Could you check a few things on this model? Use its own coordinates, in mm. Coordinates: 2 decimals unless noted, no trailing zeros. Write each loop counter-clockwise with the first axis right and the second up, starting at its lowest first coordinate (ties: lowest second). Pieces come first, ordered by that corner, then holes.
Item 1: I want a section at C-C on x = -134. Please give me the cut outline in (y, z) (3 decimals), then the cut area to 4 significant figures.
Item 2: For P1, Ø5.5, axis at x = -134, y = 105, coming from the -Z side, with a flat end and sliding along its axis, tell me the tip position at first contact or that it passes through.
Item 3: I want a section at A-A on y = 80. Please give me the cut outline in (x, z) (3 decimals), then the cut area to 4 significant figures.
Item 4: If I drill on probe 1 along X at (y, z) = (28, 0.35); probe 2 along Y at (x, z) = (-5, 0.35) (3 decimals); probe 3 along X at (y, z) = (29, 0.15), over which ranges is the centre line in solid material (lowest first)?
Item 5: I want a section at B-B on z = 0.2. State how many separate pieces and enclosed holes the cut face has, then the cut area to 3 significant figures.
from build123d import *

# Parameters (mm, degrees)
RESSALTO_EXTRUS_O1_DEPTH                       = 0.5
BROCA_DE_ROSQUEAR_PARA_TARRAXA_DE_M3X0_5_D     = 6.35
BROCA_DE_ROSQUEAR_PARA_TARRAXA_DE_M3X0_5_DEPTH = 23.492267535
BROCA_DE_ROSQUEAR_PARA_TARRAXA_DE_M3X0_5_TIP   = 1.907732465


with BuildPart() as part:
    # Esboço1 → Ressalto-extrusão1 (new body)
    with BuildSketch(Plane.XY):
        with BuildLine():
            Line((-10, 0), (-164, 0))
            ThreePointArc((-164, 0), (-171.071067812, 2.928932188), (-174, 10))
            Line((-174, 10), (-174, 100))
            ThreePointArc((-174, 100), (-171.071067812, 107.071067812), (-164, 110))
            Line((-164, 110), (-10, 110))
            ThreePointArc((-10, 110), (-2.928932188, 107.071067812), (0, 100))
            Line((0, 100), (0, 10))
            ThreePointArc((0, 10), (-2.928932188, 2.928932188), (-10, 0))
        make_face()
    extrude(amount=RESSALTO_EXTRUS_O1_DEPTH)

    # Broca de rosquear para tarraxa de M3x0.51
    with Locations(Plane.XY.offset(0.5)):
        with Locations((-169, 80), (-134, 105), (-40, 105), (-5, 80), (-5, 30), (-169, 30), (-134, 5), (-40, 5)):
            Hole(BROCA_DE_ROSQUEAR_PARA_TARRAXA_DE_M3X0_5_D / 2, depth=BROCA_DE_ROSQUEAR_PARA_TARRAXA_DE_M3X0_5_DEPTH)
            with Locations((0, 0, -(BROCA_DE_ROSQUEAR_PARA_TARRAXA_DE_M3X0_5_DEPTH + BROCA_DE_ROSQUEAR_PARA_TARRAXA_DE_M3X0_5_TIP / 2))):  # 118° drill point
                Cone(0, BROCA_DE_ROSQUEAR_PARA_TARRAXA_DE_M3X0_5_D / 2, BROCA_DE_ROSQUEAR_PARA_TARRAXA_DE_M3X0_5_TIP, mode=Mode.SUBTRACT)


solid = part.part
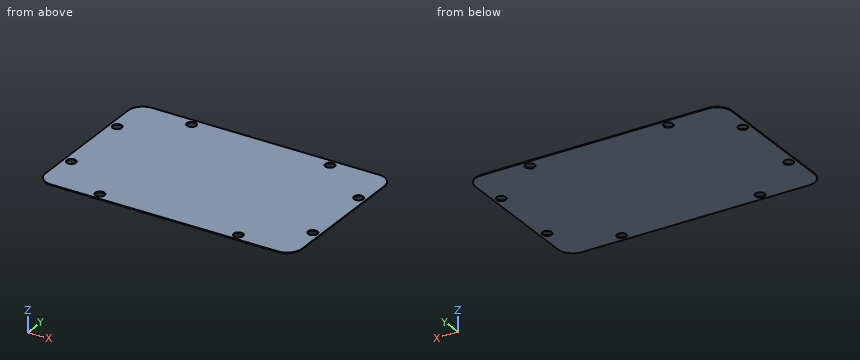
Response values:
1. outline: (0, 0) - (1.825, 0) - (1.825, 0.5) - (0, 0.5) - close; (8.175, 0) - (101.825, 0) - (101.825, 0.5) - (8.175, 0.5) - close; (108.175, 0) - (110, 0) - (110, 0.5) - (108.175, 0.5) - close
1. area: 48.65 mm2
2. P1: passes through
3. outline: (-174, 0) - (-172.175, 0) - (-172.175, 0.5) - (-174, 0.5) - close; (-165.825, 0) - (-8.175, 0) - (-8.175, 0.5) - (-165.825, 0.5) - close; (-1.825, 0) - (0, 0) - (0, 0.5) - (-1.825, 0.5) - close
3. area: 80.65 mm2
4. probe 1: x = -174 to -171.47, -166.53 to -7.47, -2.53 to 0
4. probe 2: y = 1.34 to 26.825, 33.175 to 76.825, 83.175 to 108.66
4. probe 3: x = -174 to -172.01, -165.99 to -8.01, -1.99 to 0
5. separate pieces: 1
5. enclosed holes: 8
5. area: 18,800 mm2
